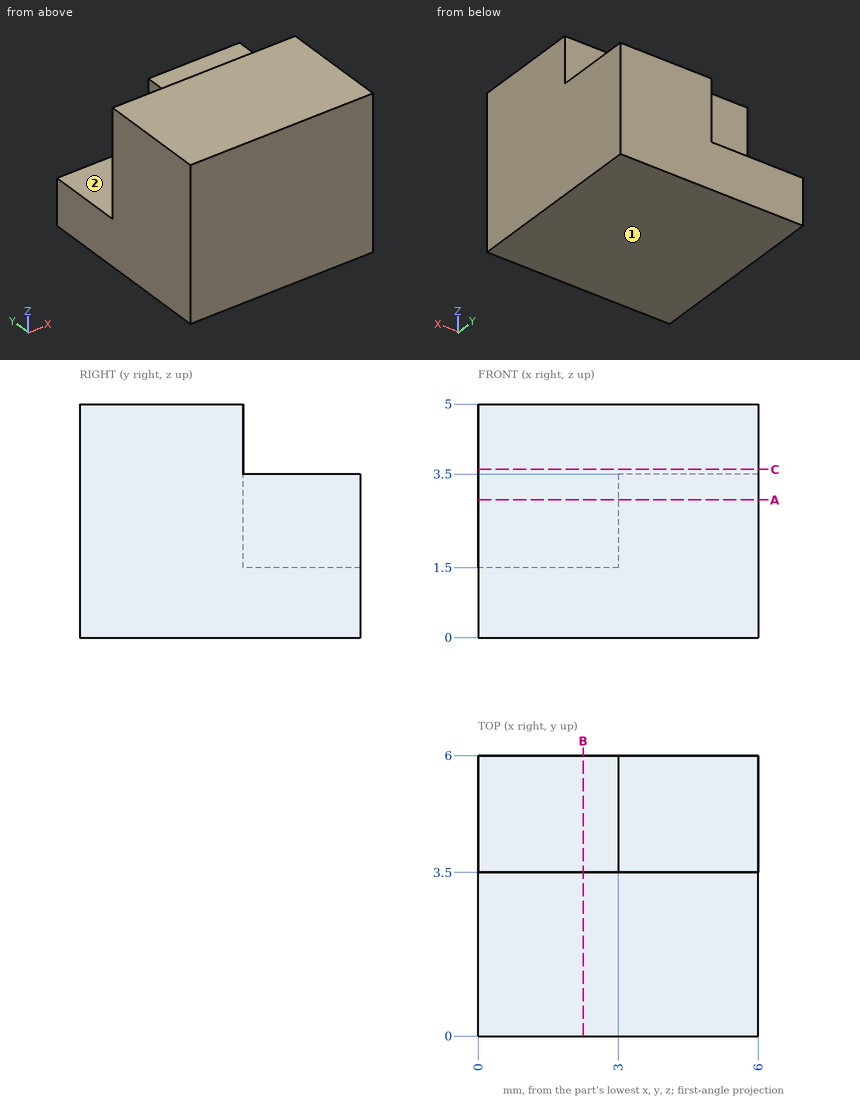
Design review of the part shown in the three views and the two pictorial views. Dimensions are in mm from the part's minimum x, y and z. A direction names the side the tool comes from. Round coordinates to 2 decimals unless told otherwise and drop trailing zeros. Write each loop counter-clockwise with the first axis right and the second up, starting at its lowest first coordinate (ties: lowest second). Pieces come first, ordered by that corner, then holes. Notation, with made-up numbers: (87, 30) -> (133, 30) arc R24 ccw to (133, 55) -> close; hole circle Ø9 at (35.25, 73.5). An arc over 180 degrees is marked (long way). Use one line per item in the form item = value.
1) Clearance check with a flat-ended pin moving along its axis: pin 1 (3 mm diameter, centred on x = 2, y = 3, fed in from -Z). State where the tip first meets the part, or that it passes through.
Found:
pin_1 = 0
2) Tool access review of the marked faces 1 and 2: name each direction out of +Z, -Z, +X, -X, +Y, -Y from which nothing blocks a thin tool from reaching the whole face with its end or side.
Found:
face_1 = -Z, +X, -X, +Y, -Y
face_2 = +Z, -X, +Y
3) Take a section at A-A, the plane z = 2.95. Write out the cut boundary in (x, y), and give its area (3 significant figures).
Found:
outline = (0, 0) -> (6, 0) -> (6, 6) -> (3, 6) -> (3, 3.5) -> (0, 3.5) -> close
area = 28.5 mm2
4) Take a section at B-B, the plane x = 2.25. Write out the cut boundary in (y, z), and give its area (4 significant figures).
Found:
outline = (0, 0) -> (6, 0) -> (6, 1.5) -> (3.5, 1.5) -> (3.5, 5) -> (0, 5) -> close
area = 21.25 mm2
5) Take a section at C-C, the plane z = 3.6. Write out the cut boundary in (x, y).
Found:
outline = (0, 0) -> (6, 0) -> (6, 3.5) -> (0, 3.5) -> close
6) To check wall thickness, follow L1, parallel to Y at x = 1.45, z = 2.65; L2, parallel to X at y = 5.4, z = 3.35. State the ranges of each line that lie inside material, in increasing order. Write a range as from..to.
Found:
L1 = 0..3.5
L2 = 3..6
